Input: part model. Units: mm. Frame: model coordinates. Give positions to 0.01 mm unless a question says otherwise; leave off trailing zeros. Loops run counter-clockwise (first coordinate to the right, second up) from the corner with the lowest first, then second, coordinate; pieces in that order, holes last. Notation, with made-up numbers: (47, -6.75) - (94, -6.75) arc R18 ccw to (94, 21.25) - close; hole circle Ø7 at (56, 88). An arc over 180 degrees is marked (long way). Answer as a JSON object with one key per item and string values. Group by question number.
(1) Mould query, pull axis Y, two halves, no side actions, for faces 1 (the cylindrical face through (0.36, -159.92, 30.58)), 2 (the flat face through (0, -177.8, 49)), 3 (the flat face through (25.4, -107, 14)). Classes: +Y half, -Y half, draft (parallel to the pull), parting line (faces both ways), or undercut.
(2) Pin query (flat end, axial travel): P1, Ø1, axis at x = 11.5, y = -33.5, coming from the -Z side; P2, Ø1.5, axis at x = -5.5, y = -75, coming from the +Z side; P3, Ø1, axis at x = -3, z = 23.5, coming from the -Y side; P4, Ø2, axis at y = -120.5, z = 26.5, coming from the +X side. Return the tip coordinate at first contact, or that it passes through.
(3) Section query B-B (y = -82). Return loops of the section in (x, z) (3 decimals).
(4) Material intervals for L1, parallel to Y at x = 8.5, z = 56.5; L2, parallel to Z at x = -18, y = -21; L3, parallel to Z at x = 10, y = -26, sorted ascending.
(5) Section query C-C (z = 34.5). Return loops of the section in (x, y), plus the area to 3 significant figures.
(6) Section query A-A (x = 0). Return loops of the section in (y, z).
```python
from build123d import *

# Parameters (mm, degrees)
F1_DEPTH = 139.7
F2_W     = 50.8
F2_H     = 52.107124
F3_DEPTH = 38.1
F5_DEPTH = 50.8


with BuildPart() as f1:
    # F0 (on Front) → F1 (new body)
    with BuildSketch(Plane.XZ):
        with BuildLine():
            Line((-25.4, 0), (0, 0))
            Line((0, 0), (25.4, 0))
            Line((25.4, 0), (25.4, 15.875))
            Line((25.4, 15.875), (21.106379, 15.875))
            ThreePointArc((21.106379, 15.875), (0, 50.741647), (-21.106379, 15.875))
            Line((-21.106379, 15.875), (-25.4, 15.875))
            Line((-25.4, 15.875), (-25.4, 0))
        make_face()
    extrude(amount=F1_DEPTH)

    # F2 (on face) → F3 (join)
    with BuildSketch(Plane.XZ.offset(139.7)):
        with BuildLine():
            Line((-25.4, 52.107124), (25.4, 52.107124))
            ThreePointArc((25.4, 52.107124), (0, 59.583701), (-25.4, 52.107124))
        make_face()
        with Locations((0, 26.053562)):
            Rectangle(F2_W, F2_H)
    extrude(amount=F3_DEPTH)

    # F4 (on face) → F5 (cut)
    with BuildSketch(Plane.YZ.offset(25.4)):
        with BuildLine():
            Line((-177.8, 42.519599), (-177.8, 19.3548))
            ThreePointArc((-177.8, 19.3548), (-159.914738, 30.937199), (-177.8, 42.519599))
        make_face()
    extrude(amount=-F5_DEPTH, mode=Mode.SUBTRACT)


solid = f1.part
```
Recorded:
{
 "1": {"face 1": "undercut", "face 2": "-Y half", "face 3": "draft"},
 "2": {"P1": "stops at z = 0", "P2": "stops at z = 50.26", "P3": "stops at y = -162.7", "P4": "stops at x = 23.82"},
 "3": {"outline": "(-25.4, 0) - (25.4, 0) - (25.4, 15.875) - (21.106, 15.875) arc R23.822 ccw (long way) to (-21.106, 15.875) - (-25.4, 15.875) - close"},
 "4": {"L1": "y = -177.8 to -139.7", "L2": "z = 0 to 42.52", "L3": "z = 0 to 48.54"},
 "5": {"outline": "(-25.4, -160.43) - (25.4, -160.43) - (25.4, -139.7) - (22.58, -139.7) - (22.58, 0) - (-22.58, 0) - (-22.58, -139.7) - (-25.4, -139.7) - close", "area": "7,360 mm^2"},
 "6": {"outline": "(-177.8, 0) - (0, 0) - (0, 50.74) - (-139.7, 50.74) - (-139.7, 59.58) - (-177.8, 59.58) - (-177.8, 42.52) arc R12.69 cw (long way) to (-177.8, 19.35) - close"}
}
